For this review, take the finished solid that the model builds, in its own axes (mm). A direction names the side the tool comes from. Coordinates: 2 decimals unless noted, no trailing zeros. Loops run counter-clockwise (first coordinate to the right, second up) from the corner with the lowest first, then second, coordinate; pieces in that order, holes last. Notation, with made-up numbers: (39, -4) - (55, -4) arc R32 cw to (55, 27) - close; hole circle Ø11 at (66.5, -39). An arc over 180 degrees is marked (long way). Answer as a JSON object with one key per item and string values. Group by question number.
Item 1: Tool access review of faces 1 (the flat face through (-53, 3, -7.938)), 2 (the flat face through (7.938, 3, -59)), 3 (the flat face through (-79.375, 3, 0)): name each direction out of +Z, -Z, +X, -X, +Y, -Y from which nothing blocks a thin tool from reaching the whole face with its end or side.
Item 2: Mouldability with a two-part tool opening along Z and no side actions: class faces 4 (the cylindrical face through (-20.1, 3.13, -20.31)), 5 (the flat face through (-58, 3, 7.937)), 6 (the cylindrical face through (-10.11, 3.13, -10.54)) as released by +Z, released by -Z, zero draft, split by the parting line, or undercut.
Item 3: To check wall thickness, follow line 1 (Z direction, x = -69.85, y = 5); line 2 (Z direction, x = -67, y = 3.5). State the ranges of each line that lie inside material, in increasing order.
Item 4: We need section C-C (y = 1). State how many separate pieces and enclosed holes the cut face has, then the cut area to 3 significant figures.
Item 5: We need section A-A (z = -69.85). Give the boundary of the cut face in (x, y).
Item 6: We need section B-B (x = -69.85). Give the boundary of the cut face in (y, z).
Item 7: Clearance check with flat-ended pins moving along their axes: pin 1 (3 mm diameter, centred on y = 2.5, z = 7.5, fed in from +X); pin 2 (1 mm diameter, centred on x = -4.5, y = 1, fed in from -Z); pin 3 (3 mm diameter, centred on y = 3.5, z = -54, fed in from -X). State where each tip first meets the part, or that it passes through.
Item 8: We need section D-D (x = -56.5). Give the boundary of the cut face in (y, z).
from build123d import *

# Parameters (mm, degrees)
SKETCH1_R                    = 28.575
SKETCH1_R_2                  = 14.605
BOSS_EXTRUDE1_DEPTH          = 6.35
BOSS_EXTRUDE2_DEPTH          = 6.35
F_0_257_DIAMETER_HOLE1_D     = 6.5278
CIRPATTERN1_COUNT            = 4
CUT_EXTRUDE1_DEPTH           = 113.432663181
FILLET1_R                    = 6.35
BOSS_EXTRUDE3_DEPTH          = 6.35
F_18_0_1695_DIAMETER_HOLE1_D = 4.3053
FILLET2_R                    = 6.35


with BuildPart() as part:
    # Sketch1 → Boss-Extrude1 (new body)
    with BuildSketch(Plane(origin=(0, 0, 0), x_dir=(1, 0, 0), z_dir=(0, 1, 0))):
        with Locations(Location((0, 0, 0), (0, 0, 270))):
            Circle(SKETCH1_R)
        with Locations(Location((0, 0, 0), (0, 0, 270))):
            Circle(SKETCH1_R_2, mode=Mode.SUBTRACT)
    extrude(amount=BOSS_EXTRUDE1_DEPTH)

    # Sketch2 → Boss-Extrude2 (add)
    with BuildSketch(Plane(origin=(0, 6.35, 0), x_dir=(1, 0, 0), z_dir=(0, 1, 0))):
        with BuildLine():
            Line((73.025, -7.9375), (25.4, -7.9375))
            Line((25.4, -7.9375), (25.4, 7.9375))
            Line((25.4, 7.9375), (73.025, 7.9375))
            ThreePointArc((73.025, 7.9375), (77.515128061, 6.077628061), (79.375, 1.5875))
            Line((79.375, 1.5875), (79.375, -1.5875))
            ThreePointArc((79.375, -1.5875), (77.515128061, -6.077628061), (73.025, -7.9375))
        make_face()
    boss_extrude2 = extrude(amount=-BOSS_EXTRUDE2_DEPTH)

    # F (0.257) Diameter Hole1 (through all)
    with Locations(Plane(origin=(0, 6.35, 0), x_dir=(1, 0, 0), z_dir=(0, 1, 0))):
        with Locations((69.85, 0)):
            f_0_257_diameter_hole1 = Hole(F_0_257_DIAMETER_HOLE1_D / 2)

    # CirPattern1: Boss-Extrude2, F (0.257) Diameter Hole1 ×4 about axis
    cirpattern1_axis = Axis((0, 0, 0), (0, 1, 0))
    add([boss_extrude2.rotate(cirpattern1_axis, i * 360 / CIRPATTERN1_COUNT) for i in range(1, CIRPATTERN1_COUNT)])
    add([f_0_257_diameter_hole1.rotate(cirpattern1_axis, i * 360 / CIRPATTERN1_COUNT) for i in range(1, CIRPATTERN1_COUNT)], mode=Mode.SUBTRACT)

    # Sketch5 → Cut-Extrude1 (cut, through all)
    with BuildSketch(Plane(origin=(0, 6.35, 0), x_dir=(1, 0, 0), z_dir=(0, 1, 0))):
        Polygon((-38.294182992, -36.049118961), (36.049118961, 38.294182992), (38.294182992, 36.049118961), (-36.049118961, -38.294182992), align=None)
    extrude(amount=-CUT_EXTRUDE1_DEPTH, mode=Mode.SUBTRACT)


with BuildPart() as body_2:
    # of the pieces the cut leaves, the one that is kept (cut_extrude1_keep)
    add(part.part.solids().sort_by_distance((19.051838715, 0, -21.296902746))[0])

    # Fillet1
    fillet1_edges = [body_2.edges().sort_by_distance(p)[0] for p in [
        (-7.9375, 3.175, -27.450441139),
        (-27.450441139, 3.175, -7.9375),
    ]]
    fillet(fillet1_edges, radius=FILLET1_R)

    # Sketch7 → Boss-Extrude3 (add)
    with BuildSketch(Plane(origin=(0, 6.35, 0), x_dir=(1, 0, 0), z_dir=(0, 1, 0))):
        Polygon((-14.513140303, -12.268076272), (-25.738460454, -23.493396424), (-45.944036726, -3.287820151), (-34.718716575, 7.9375), align=None)
    boss_extrude3 = extrude(amount=-BOSS_EXTRUDE3_DEPTH)

    # #18 (0.1695) Diameter Hole1 (through all)
    with Locations(Plane(origin=(0, 6.35, 0), x_dir=(1, 0, 0), z_dir=(0, 1, 0))):
        with Locations((-30.228588515, -10.023012242), (-39.208844636, -1.042756121)):
            f_18_0_1695_diameter_hole1 = Hole(F_18_0_1695_DIAMETER_HOLE1_D / 2)

    # Mirror1: Boss-Extrude3, #18 (0.1695) Diameter Hole1 across plane
    add(boss_extrude3.mirror(Plane(origin=(0, 0, 0), x_dir=(0.7071067811865478, 0, 0.7071067811865472), z_dir=(0.7071067811865475, 0, -0.7071067811865477))))
    add(f_18_0_1695_diameter_hole1.mirror(Plane(origin=(0, 0, 0), x_dir=(0.7071067811865478, 0, 0.7071067811865472), z_dir=(0.7071067811865475, 0, -0.7071067811865477))), mode=Mode.SUBTRACT)

    # Fillet2
    fillet2_edges = [body_2.edges().sort_by_distance(p)[0] for p in [
        (-41.294356878, 3.175, 7.9375),
        (7.9375, 3.175, -41.294356878),
    ]]
    fillet(fillet2_edges, radius=FILLET2_R)


solid = body_2.part
Check sheet entries:
{
 "1": {"face 1": "-Z, -X, +Y, -Y", "face 2": "-Z, +X, +Y, -Y", "face 3": "+Z, -Z, -X, +Y, -Y"},
 "2": {"face 4": "released by -Z", "face 5": "released by +Z", "face 6": "undercut"},
 "3": {"line 1": "z = -7.94 to -3.26, 3.26 to 7.94", "line 2": "z = -7.94 to -1.59, 1.59 to 7.94"},
 "4": {"separate pieces": "1", "enclosed holes": "6", "area": "2,660 mm2"},
 "5": {"outline": "(-7.94, 0) - (-3.26, 0) - (-3.26, 6.35) - (-7.94, 6.35) - close; (3.26, 0) - (7.94, 0) - (7.94, 6.35) - (3.26, 6.35) - close"},
 "6": {"outline": "(0, -7.94) - (6.35, -7.94) - (6.35, -3.26) - (0, -3.26) - close; (0, 3.26) - (6.35, 3.26) - (6.35, 7.94) - (0, 7.94) - close"},
 "7": {"pin 1": "stops at x = -11.5", "pin 2": "stops at z = -78.9", "pin 3": "stops at x = -7.94"},
 "8": {"outline": "(0, -7.94) - (6.35, -7.94) - (6.35, 7.94) - (0, 7.94) - close"}
}
